from build123d import *

# Parameters (mm, degrees)
SKETCH1_R           = 9
SKETCH1_R_2         = 2.675
BOSS_EXTRUDE1_DEPTH = 16.98
SKETCH2_R           = 10.875
SKETCH2_R_2         = 2.675
BOSS_EXTRUDE2_DEPTH = 7
SKETCH4_R           = 9
SKETCH4_R_2         = 2.675
BOSS_EXTRUDE3_DEPTH = 7.5


with BuildPart() as part:
    # Sketch1 → Boss-Extrude1 (new body)
    with BuildSketch(Plane.XY):
        Circle(SKETCH1_R)
        Circle(SKETCH1_R_2, mode=Mode.SUBTRACT)
    extrude(amount=BOSS_EXTRUDE1_DEPTH)

    # Sketch2 → Boss-Extrude2 (add)
    with BuildSketch(Plane.XY.offset(16.98)):
        Circle(SKETCH2_R)
        Circle(SKETCH2_R_2, mode=Mode.SUBTRACT)
    extrude(amount=BOSS_EXTRUDE2_DEPTH)

    # Sketch4 → Boss-Extrude3 (add)
    with BuildSketch(Plane.XY.offset(23.98)):
        Circle(SKETCH4_R)
        Circle(SKETCH4_R_2, mode=Mode.SUBTRACT)
    extrude(amount=BOSS_EXTRUDE3_DEPTH)


solid = part.part
Could you check a few things on this model? Use its own coordinates, in mm. A direction names the side the tool comes from. Coordinates: 2 decimals unless noted, no trailing zeros. Write each loop counter-clockwise with the first axis right and the second up, starting at its lowest first coordinate (ties: lowest second). Pieces come first, ordered by that corner, then holes. Notation, with made-up numbers: (24.5, 4) - (37.5, 4) arc R23 ccw to (37.5, 36) - close; hole circle Ø11 at (-11, -9). An arc over 180 degrees is marked (long way). Write item = value, one per line.
1) Please list where these lines run through material, in increasing order: line 1 (Y direction, x = 0, z = 23.5) (3 decimals); line 2 (Y direction, x = 0, z = 25) (3 decimals); line 3 (Z direction, x = 3.25, y = 9.5). Write a range as [from, to].
Result set:
line_1 = [-10.875, -2.675], [2.675, 10.875]
line_2 = [-9, -2.675], [2.675, 9]
line_3 = [16.98, 23.98]
2) Will these pins go through, and if not, where does the flat tip stop? pin 1 Ø1 at (y, z) = (-8.5, 8) entering from +X; pin 2 Ø1.5 at (y, z) = (2.5, 4) entering from -X; pin 3 Ø1 at (y, z) = (-2, 13) entering from -X; pin 4 Ø4 at (x, y) = (-6, -0.5) entering from -Z.
Result set:
pin_1 = 4.12
pin_2 = -8.83
pin_3 = -8.87
pin_4 = 0
3) We'd pull the mould along Y, two halves only. Please class faces 1 (the flat face through (2, 9, 16.98)), 2 (the cylindrical face through (-1.42, 10.78, 20.43)), 3 (the cylindrical face through (-0.58, -2.61, 15.52)): +Y half, -Y half, draft (parallel to the pull), parting line (faces both ways), or undercut.
Result set:
face_1 = draft
face_2 = parting line
face_3 = undercut
4) Suppose I cut it at A-A on x = 0. Please give me the cut outline in (y, z) (3 decimals), plus the area to 3 significant figures.
Result set:
outline = (-10.875, 16.98) - (-9, 16.98) - (-9, 0) - (-2.675, 0) - (-2.675, 31.48) - (-9, 31.48) - (-9, 23.98) - (-10.875, 23.98) - close; (2.675, 0) - (9, 0) - (9, 16.98) - (10.875, 16.98) - (10.875, 23.98) - (9, 23.98) - (9, 31.48) - (2.675, 31.48) - close
area = 424 mm2
5) For faces 4 (the cylindrical face through (-1.172, 8.923, 8.371)), 5 (the flat face through (-2, -2, 0)), 6 (the cylindrical face through (-1.172, 8.923, 27.678)), which set-ups out of +Z, -Z, +X, -X, +Y, -Y let a thin tool reach every point of the face, with its end or its side?
Result set:
face_4 = -Z
face_5 = -Z, +X, -X, +Y, -Y
face_6 = +Z
6) Suppose I cut it at D-D on x = 6. Please give me the cut outline in (y, z).
Result set:
outline = (-9.07, 16.98) - (-6.71, 16.98) - (-6.71, 0) - (6.71, 0) - (6.71, 16.98) - (9.07, 16.98) - (9.07, 23.98) - (6.71, 23.98) - (6.71, 31.48) - (-6.71, 31.48) - (-6.71, 23.98) - (-9.07, 23.98) - close
7) Suppose I cut it at C-C on z = 19. Please give me the cut outline in (x, y) (3 decimals).
Result set:
outline = circle Ø21.75 at (0, 0); hole circle Ø5.35 at (0, 0)
